The listing builds one solid part. Answer for the finished solid, in the listing's coordinates (mm). Face numbers are marked on the shaded views. Coordinates: 2 decimals unless noted, no trailing zeros. Write each loop counter-clockwise with the first axis right and the second up, starting at its lowest first coordinate (ties: lowest second). Pieces come first, ordered by that corner, then holes.
```python
from build123d import *

# Parameters (mm, degrees)
CHAMFER1_SIZE = 0.762
FILLET1_R     = 1.524
FILLET2_R     = 0.762


with BuildPart() as part:
    # Sketch1 → Revolve1 (revolve)
    with BuildSketch(Plane.XY, mode=Mode.PRIVATE) as revolve1_sk:
        with BuildLine():
            Line((0, 0), (-9.525, 0))
            Line((-9.525, 0), (-9.525, 3.175))
            Line((-9.525, 3.175), (-8.001, 3.175))
            Line((-8.001, 3.175), (-8.001, 4.699))
            Line((-8.001, 4.699), (-6.477, 4.699))
            Line((-6.477, 4.699), (-5.3848, 28.6766))
            Line((-5.3848, 28.6766), (-6.2484, 28.6766))
            Line((-6.2484, 28.6766), (-6.2484, 30.2006))
            Line((-6.2484, 30.2006), (-4.7244, 30.2006))
            Line((-4.7244, 30.2006), (-4.7244, 31.7246))
            Line((-4.7244, 31.7246), (-3.9624, 31.7246))
            Line((-3.9624, 31.7246), (-6.2484, 39.624))
            Line((-6.2484, 39.624), (-4.6228, 39.116))
            Line((-4.6228, 39.116), (-0.569581457, 40.006817262))
            ThreePointArc((-0.569581457, 40.006817262), (-0.695109792, 40.825196055), (0, 41.275))
            Line((0, 41.275), (0, 0))
        make_face()
    revolve(revolve1_sk.sketch.rotate(Axis((0, 0, 0), (0, 1, 0)), 270), axis=Axis((0, 0, 0), (0, 1, 0)))

    # Chamfer1
    chamfer1_edges = [part.edges().sort_by_distance(p)[0] for p in [
        (0, 3.175, 9.525),
        (0, 31.7246, 4.7244),
    ]]
    chamfer(chamfer1_edges, length=CHAMFER1_SIZE - 0.0001)  # a hair under: the kernel refuses the full size

    # Fillet1
    fillet1_edges = [part.edges().sort_by_distance(p)[0] for p in [
        (0, 4.699, 8.001),
    ]]
    fillet(fillet1_edges, radius=FILLET1_R - 0.0001)  # a hair under: the kernel refuses the full size

    # Fillet2
    fillet2_edges = [part.edges().sort_by_distance(p)[0] for p in [
        (0, 28.6766, 6.2484),
        (0, 30.2006, 6.2484),
    ]]
    fillet(fillet2_edges, radius=FILLET2_R - 0.0001)  # a hair under: the kernel refuses the full size


solid = part.part
```
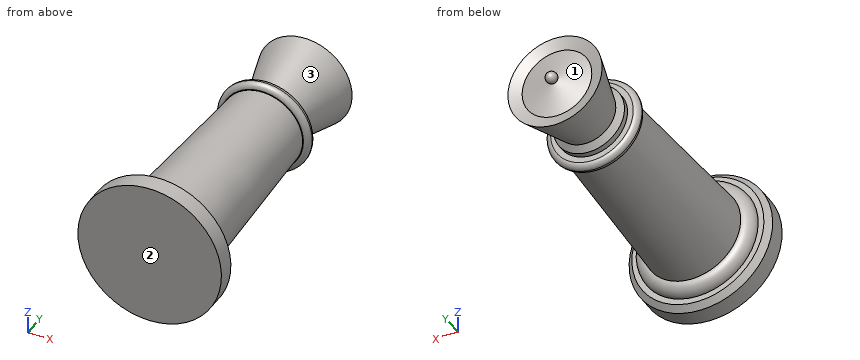
(1) For a pull along X with two mould halves and no side action, classify the marked faces 1, 2 and 3 as pulls with the +X half, pulls with the -X half, needs draft (parallel to the pull), parting line crosses it, or undercut.
(2) Each of these flat-tipped pins is pushed along its axis until it touches: pin 1 (9 mm diameter, centred on x = -0.5, z = -0.5, fed in from -Y); pin 2 (3 mm diameter, centred on x = -2.5, y = 33.5, fed in from -Z); pin 3 (6 mm diameter, centred on x = -6.5, y = 17.5, fed in from +Z); pin 4 (4 mm diameter, centred on y = 9, z = -2, fed in from -X). Where does it stop, or does it pass through?
(3) Find the intervals of material crossed by probe 1 along Y at (x, z) = (-3.25, -5.75); probe 2 along Z at (x, y) = (2.5, 31); probe 3 along Y at (x, z) = (8.25, 0.5) (3 decimals), in increasing order.
(4) Section B-B, the plane y = 36 is taken. Write down the section's boundary in (x, z).
(5) Section A-A, the plane y = 27 is taken. Write down the section's boundary in (x, z), plus the area to 3 significant figures.
Solution:
1. face 1: undercut
1. face 2: needs draft
1. face 3: parting line crosses it
2. pin 1: stops at y = 0
2. pin 2: stops at z = -4.56
2. pin 3: stops at z = 4.75
2. pin 4: stops at x = -6.32
3. probe 1: y = 0 to 4.69
3. probe 2: z = -3.96 to 3.96
3. probe 3: y = 0 to 3.175
4. outline: circle Ø10.4 at (0, 0)
5. outline: circle Ø10.92 at (0, 0)
5. area: 93.7 mm2
